Could you check a few things on this drawing? It's one solid part, dimensions in mm from its lowest x, y, z. A direction names the side the tool comes from. Give positions to 0.01 mm unless a question says otherwise; leave off trailing zeros. Loops run counter-clockwise (first coordinate to the right, second up) from the corner with the lowest first, then second, coordinate; pieces in that order, holes last. Notation, with made-up numbers: M 43.5,65 L 57.5,65 A18 ccw 57.5,81 Z; hole C 71.25,-8.5 d1. An arc over 180 degrees is marked long. Return JSON: item names as keys, results as strings. Group by question number.
1. If we mould it in two halves opening along Z, with no side actions, what happens to the marked faces 5, 6 and 7? For each: +Z half, -Z half, draft (parallel to the pull), parting line (faces both ways), or undercut.
2. For pin 1 (3 mm diameter, centred on y = 60.5, z = 62, fed in from -X); pin 2 (5 mm diameter, centred on y = 12, z = 20, fed in from +X); pin 3 (1.2 mm diameter, centred on x = 84, y = 49, fed in from +Z), each with a flat end and sliding along its axis, tell me the tip position at first contact or that it passes through.
3. If we section it at A-A (x = 34): Write out the boundary of the cut face in (y, z).
4. If we section it at D-D (x = 112): Write out the boundary of the cut face in (y, z), plus the area to 3 significant figures.
5. Please list where these lines run through material, in increasing order: line 1 (Y direction, x = 46, z = 67.5); line 2 (X direction, y = 63, z = 21); line 3 (Z direction, x = 79, y = 23).
6. If we section it at C-C (y = 20.5): Write out the boundary of the cut face in (x, z).
7. For the marked faces 1, 2, 3 and 4, which set-ups out of +Z, -Z, +X, -X, +Y, -Y let a thin tool reach every point of the face, with its end or its side?
8. If we section it at B-B (z = 19): Write out the boundary of the cut face in (x, y), plus the area to 3 significant figures.
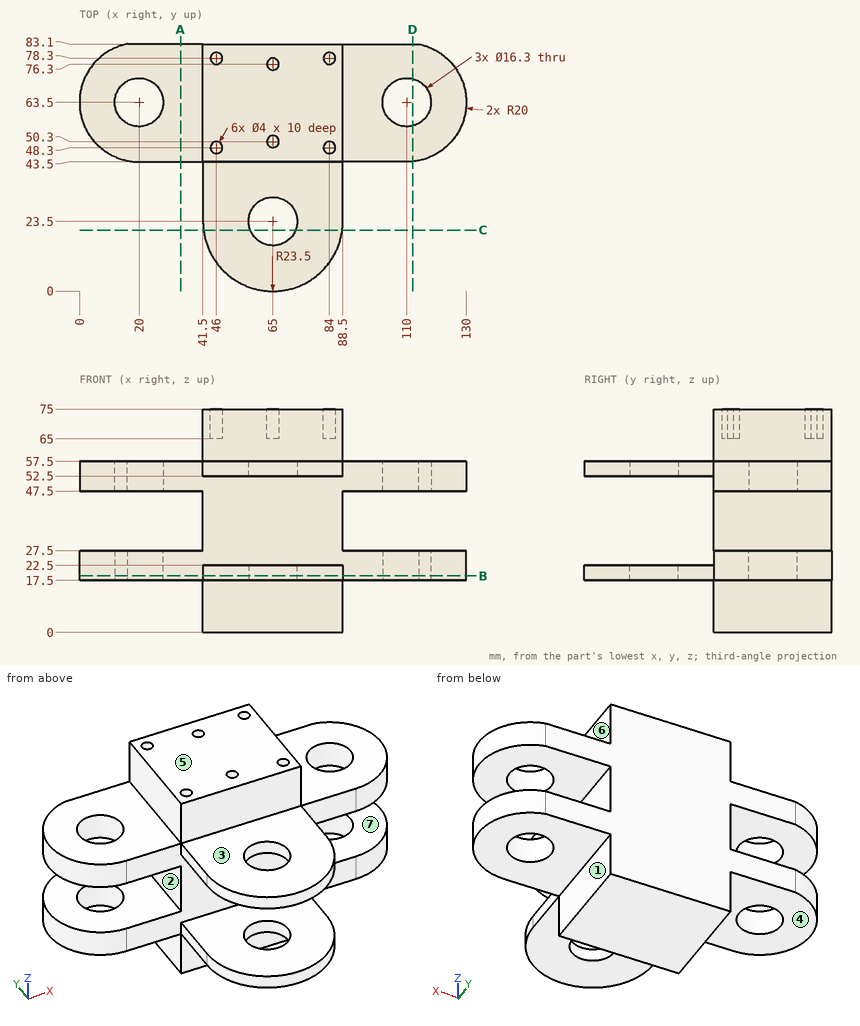
Answer:
{
 "1": {"face 5": "+Z half", "face 6": "draft", "face 7": "undercut"},
 "2": {"pin 1": "stops at x = 41.5", "pin 2": "stops at x = 86.71", "pin 3": "stops at z = 65"},
 "3": {"outline": "M 43.5,17.5 L 83.1,17.5 L 83.1,27.5 L 43.5,27.5 Z; M 43.5,47.5 L 83.1,47.5 L 83.1,57.5 L 43.5,57.5 Z"},
 "4": {"outline": "M 43.6,17.5 L 55.6,17.5 L 55.6,27.5 L 43.6,27.5 Z; M 43.6,47.5 L 55.6,47.5 L 55.6,57.5 L 43.6,57.5 Z; M 71.4,17.5 L 83.1,17.5 L 83.1,27.5 L 71.4,27.5 Z; M 71.4,47.5 L 83.1,47.5 L 83.1,57.5 L 71.4,57.5 Z", "area": "474 mm²"},
 "5": {"line 1": "y = 43.5 to 46.3, 50.3 to 76.3, 80.3 to 83.1", "line 2": "x = 0.01 to 11.87, 28.13 to 101.87, 118.13 to 129.99", "line 3": "z = 17.5 to 22.5, 52.5 to 57.5"},
 "6": {"outline": "M 41.69,17.5 L 57.42,17.5 L 57.42,22.5 L 41.69,22.5 Z; M 41.69,52.5 L 57.42,52.5 L 57.42,57.5 L 41.69,57.5 Z; M 72.58,17.5 L 88.31,17.5 L 88.31,22.5 L 72.58,22.5 Z; M 72.58,52.5 L 88.31,52.5 L 88.31,57.5 L 72.58,57.5 Z"},
 "7": {"face 1": "-Z, +X, +Y, -Y", "face 2": "-X, +Y, -Y", "face 3": "+Z, +X, -X, -Y", "face 4": "-Z, -X, +Y, -Y"},
 "8": {"outline": "M 16.02,83.1 A20 ccw 20,43.5 L 41.5,43.5 L 41.5,23.5 A23.5 ccw 88.5,23.5 L 88.5,43.5 L 110,43.5 A20 ccw 113.98,83.1 Z; hole C 20,63.5 d16.3; hole C 65,23.5 d16.3; hole C 110,63.5 d16.3", "area": "6,000 mm²"}
}
